Could you check a few things on this drawing? It's one solid part, dimensions in mm from its lowest x, y, z. Give positions to 0.01 mm unless a question says otherwise; leave off trailing zeros. Loops run counter-clockwise (first coordinate to the right, second up) from the corner with the lowest first, then second, coordinate; pieces in that order, holes last.
Q1. Thinking about a two-plate mould opening in Y: for the marked faces 1, 2 and 3, which applies, pulls with the +Y half, pulls with the -Y half, needs draft (parallel to the pull), parting line crosses it, or undercut?
Q2. I need wall thicknesses on probe 1 along Y at (x, z) = (142.5, 12.5); probe 2 along X at (y, z) = (184, 12.5). Which ranges of each line are inside material? Lowest first, please.
Q3. Suppose I cut it at A-A (z = 7.5). Count the separate pieces of the cut face and the enclosed holes in it, and give its area (3 significant figures).
Q4. Suppose I cut it at B-B (x = 173.5). List the corners of the cut face in (y, z) for me.
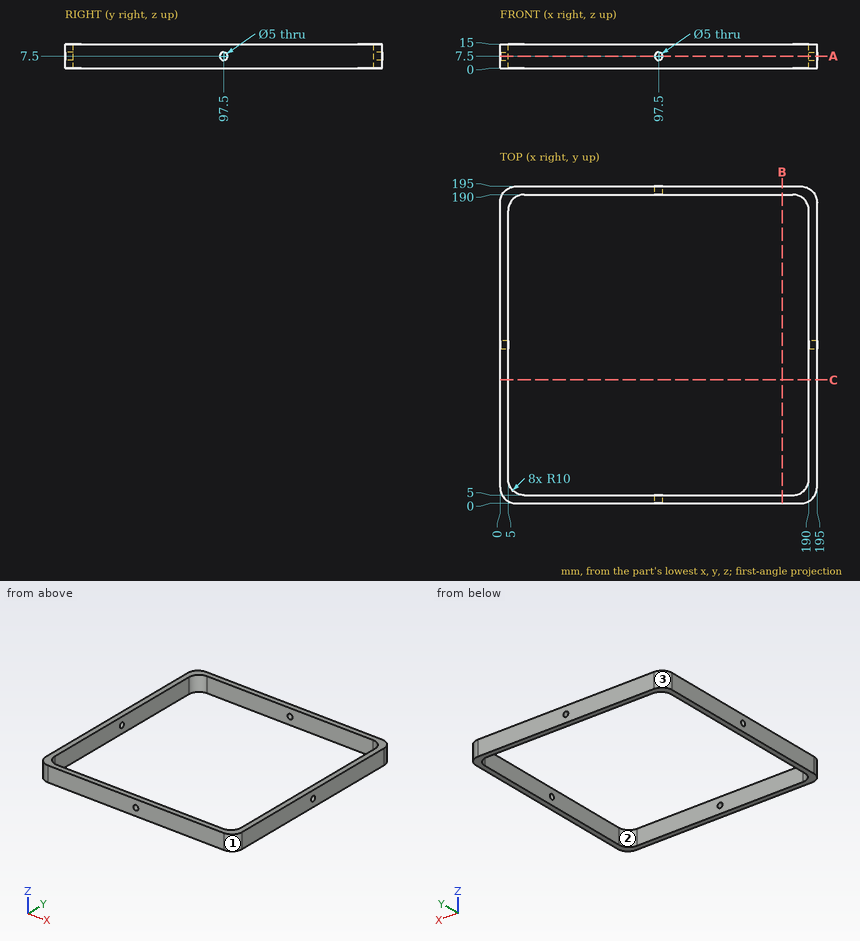
Solutions:
1. face 1: pulls with the -Y half
1. face 2: undercut
1. face 3: pulls with the +Y half
2. probe 1: y = 0 to 5, 190 to 195
2. probe 2: x = 0 to 5.83, 189.17 to 195
3. separate pieces: 4
3. enclosed holes: 0
3. area: 3,700 mm2
4. outline: (0, 0) - (5, 0) - (5, 15) - (0, 15) - close; (190, 0) - (195, 0) - (195, 15) - (190, 15) - close
